For this review, take the finished solid that the model builds, in its own axes (mm). Round coordinates to 2 decimals unless told otherwise and drop trailing zeros. Write each loop counter-clockwise with the first axis right and the second up, starting at its lowest first coordinate (ties: lowest second). Pieces come first, ordered by that corner, then holes. Notation, with made-up numbers: (56, 64) -> (94, 64) arc R9 ccw to (94, 69) -> close; hole circle Ø4 at (-34.75, 66.25). An arc over 180 degrees is marked (long way). Answer in a Markdown table with one row per item.
from build123d import *

# Parameters (mm, degrees)
F0_R     = 11.1125
F1_DEPTH = 19.05
F2_R     = 12.7
F3_R     = 2.54


with BuildPart() as f1:
    # F0 (on Front) → F1 (new body)
    with BuildSketch(Plane.XZ):
        Polygon((-15.586365, 80.178106), (-50.511365, 12.453041), (38.388635, 12.453041), (3.463635, 80.178106), align=None)
        with Locations((-6.061365, 55.315541)):
            Circle(F0_R, mode=Mode.SUBTRACT)
    extrude(amount=F1_DEPTH)

    # F2
    f2_edges = [f1.edges().sort_by_distance(p)[0] for p in [
        (-15.586365, -9.525, 80.178106),
        (3.463635, -9.525, 80.178106),
    ]]
    fillet(f2_edges, radius=F2_R)

    # F3
    f3_edges = [f1.edges().sort_by_distance(p)[0] for p in [
        (-50.511365, -9.525, 12.453041),
        (38.388635, -9.525, 12.453041),
    ]]
    fillet(f3_edges, radius=F3_R)


solid = f1.part
1) Consider section D-D on x = 12. State the section outline as (y, z) points.
Solved:
| item | result |
|---|---|
| outline | (-19.05, 12.45) -> (0, 12.45) -> (0, 63.62) -> (-19.05, 63.62) -> close |
2) For line 1 (X direction, y = -13.25, z = 59.5); line 2 (X direction, y = -2.5, z = 48.5); line 3 (Z direction, x = -3, y = -6.5), list the stretches that pass through material, from the lowest coordinate up. Write a range as [from, to].
Solved:
| item | result |
|---|---|
| line 1 | [-26.25, -16.36], [4.23, 14.13] |
| line 2 | [-31.92, -14.84], [2.72, 19.8] |
| line 3 | [12.45, 44.63], [66, 80.11] |
3) Clearance check with flat-ended pins moving along their axes: pin 1 Ø20 at (x, z) = (-6.06, 55.32) entering from +Y; pin 2 Ø10 at (y, z) = (-6.5, 71) entering from -X; pin 3 Ø4 at (y, z) = (-8.5, 48) entering from -X; pin 4 Ø4 at (y, z) = (-16, 71.5) entering from -X. State where each tip first meets the part, or that it passes through.
Solved:
| item | result |
|---|---|
| pin 1 | through |
| pin 2 | x = -22.9 |
| pin 3 | x = -33.21 |
| pin 4 | x = -21.09 |
4) Consider section A-A on z = 60.5. State the section outline as (x, y) points.
Solved:
| item | result |
|---|---|
| outline | (-25.73, -19.05) -> (-15.89, -19.05) -> (-15.89, 0) -> (-25.73, 0) -> close; (3.77, -19.05) -> (13.61, -19.05) -> (13.61, 0) -> (3.77, 0) -> close |
5) Consider section C-C on z = 75.5. State the section outline as (x, y) points.
Solved:
| item | result |
|---|---|
| outline | (-17.69, -19.05) -> (5.57, -19.05) -> (5.57, 0) -> (-17.69, 0) -> close |
6) Consider section B-B on y = -12.5. State the section outline as (x, z) points (1 decimal), then the cut area to 3 significant figures.
Solved:
| item | result |
|---|---|
| outline | (-48.6, 16.2) arc R2.5 ccw to (-46.3, 12.5) -> (34.2, 12.5) arc R2.5 ccw to (36.5, 16.2) -> (7, 73.3) arc R12.7 ccw to (-4.3, 80.2) -> (-7.8, 80.2) arc R12.7 ccw to (-19.1, 73.3) -> close; hole circle Ø22.2 at (-6.1, 55.3) |
| area | 3,240 mm² |
7) Mouldability with a two-part tool opening along Z and no side actions: class faces 1 (the cylindrical face through (-48.53, -9.66, 13.7)), 2 (the flat face through (-7, -19.05, 39)), 3 (the cylindrical face through (-0.087, -9.392, 64.686)) as pulls with the +Z half, pulls with the -Z half, needs draft (parallel to the pull), parting line crosses it, or undercut.
Solved:
| item | result |
|---|---|
| face 1 | parting line crosses it |
| face 2 | needs draft |
| face 3 | undercut |
